Autodesk Inventor part; units mm, degrees
ref_plane "YZ Plane" through (0, 0, 0) normal (1, 0, 0) x (0, 1, 0)
ref_plane "XZ Plane" through (0, 0, 0) normal (0, 1, 0) x (-1, 0, 0)
ref_plane "XY Plane" through (0, 0, 0) normal (0, 0, 1) x (1, 0, 0)
sketch "Sketch1" plane through (0, 0, 0) normal (0, 0, 1) x (1, 0, 0)
  circle A0 centre (10.5, 65) radius 2.65
  circle A1 centre (10.5, 10) radius 2.65
  circle A2 centre (49.5, 30) radius 3.5
  line L0 (0, 0) -> (60, 0)
  line L1 (60, 0) -> (60, 75)
  line L2 (60, 75) -> (0, 75)
  line L3 (0, 75) -> (0, 0)
  dimension "d0" = 39
  dimension "d1" = 5.3
  dimension "d2" = 55
  dimension "d16" = 7
  dimension "d26" = 75
  dimension "d27" = 60
  dimension "d28" = 10
  dimension "d29" = 10.5
  dimension "d32" = 20
  dimension "d44" = 10.5
  dimension "d50" = 10
extrude "Extrusion1" add sketch "Sketch1" along normal blind 6.731
fillet "Fillet1" radius 20 4 edges at (0, 75, 3.3655) (60, 75, 3.3655) (0, 0, 3.3655) (60, 0, 3.3655)
equation "\"d29\" = d44"
equation "\"d30\" = THICKB"
equation "\"THICKA\" = 3.175"
equation "\"THICKB\" = 6.731"
equation "\"THICKC\" = 12.7"
equation "\"BALLDIA\" = 12"
equation "\"MAGDIA\" = 9.5"
equation "\"THICKPLY\" = 5"
properties part number "Carriage_Frame_Back"
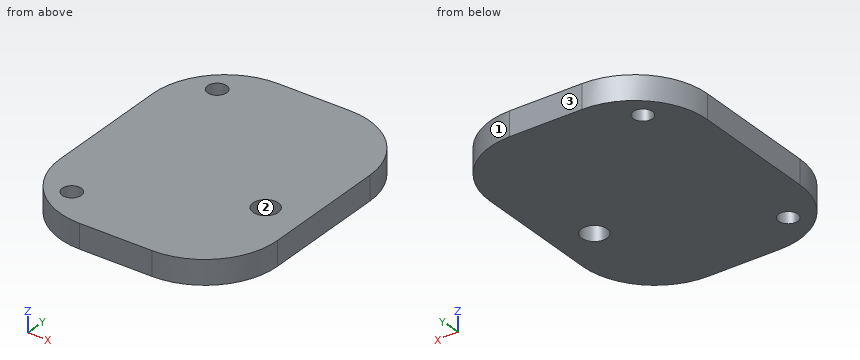
Check sheet for the modelled part. Datum: model origin and axes. Units: mm. Face numbers are marked on the shaded views. Give positions to 0.01 mm unless a question says otherwise; leave off trailing zeros. Write each loop counter-clockwise with the first axis right and the second up, starting at its lowest first coordinate (ties: lowest second). Pieces come first, ordered by that corner, then holes. Notation, with made-up numbers: M 0,71 L 5,71 A21 cw 5,90 Z; hole C -34.75,5.5 d2. An arc over 180 degrees is marked long. Use one line per item in the form item = value.
(1) Section check D-D on x = 10.5. Record the boundary of the cut face in (y, z), plus the area to 3 significant figures.
Answer block:
outline = M 2.4,0 L 7.35,0 L 7.35,6.73 L 2.4,6.73 Z; M 12.65,0 L 62.35,0 L 62.35,6.73 L 12.65,6.73 Z; M 67.65,0 L 72.6,0 L 72.6,6.73 L 67.65,6.73 Z
area = 401 mm2
(2) Material ranges on line 1 along Y through (x, z) = (10.5, 5); line 2 along X through (y, z) = (32, 3); line 3 along Y through (x, z) = (46.5, 1.25), recorded low to high.
Answer block:
line_1 = 2.4 to 7.35, 12.65 to 62.35, 67.65 to 72.6
line_2 = 0 to 46.63, 52.37 to 60
line_3 = 1.09 to 28.2, 31.8 to 73.91
(3) Draft check along X on the marked faces 1, 2 and 3. Enter one of: pulls with the +X half, pulls with the -X half, needs draft (parallel to the pull), parting line crosses it, or undercut.
Answer block:
face_1 = pulls with the +X half
face_2 = undercut
face_3 = needs draft
(4) Depth check by flat-ended pin: P1, Ø3, axis at y = 58.5, z = 4.5, coming from the +X side; P2, Ø3, axis at y = 11, z = 3, coming from the +X side; P3, Ø2, axis at x = 10, z = 2.5, coming from the -Y side; P4, Ø5.5, axis at x = 49.5, y = 30, coming from the -Z side. Enter the tip coordinate at first touch or a pass-through.
Answer block:
P1 = 59.9
P2 = 58.54
P3 = 2.14
P4 = through
(5) Section check B-B on z = 1.5. Record the boundary of the cut face in (x, y), plus the area to 3 significant figures.
Answer block:
outline = M 0,20 A20 ccw 20,0 L 40,0 A20 ccw 60,20 L 60,55 A20 ccw 40,75 L 20,75 A20 ccw 0,55 Z; hole C 10.5,10 d5.3; hole C 10.5,65 d5.3; hole C 49.5,30 d7
area = 4,070 mm2
(6) Section check C-C on x = 49.5. Record the boundary of the cut face in (y, z), plus the area to 3 significant figures.
Answer block:
outline = M 2.4,0 L 26.5,0 L 26.5,6.73 L 2.4,6.73 Z; M 33.5,0 L 72.6,0 L 72.6,6.73 L 33.5,6.73 Z
area = 425 mm2
(7) Section check A-A on y = 30. Record the boundary of the cut face in (x, z), plus the area to 3 significant figures.
Answer block:
outline = M 0,0 L 46,0 L 46,6.73 L 0,6.73 Z; M 53,0 L 60,0 L 60,6.73 L 53,6.73 Z
area = 357 mm2
